Autodesk Inventor part; units mm, degrees
ref_plane "YZ Plane" through (0, 0, 0) normal (1, 0, 0) x (0, 1, 0)
ref_plane "XZ Plane" through (0, 0, 0) normal (0, 1, 0) x (-1, 0, 0)
ref_plane "XY Plane" through (0, 0, 0) normal (0, 0, 1) x (1, 0, 0)
sketch "Sketch1" plane through (0, 0, 0) normal (0, 0, 1) x (1, 0, 0)
  circle A0 centre (0, 0) radius 2.3813
  circle A1 centre (0, 0) radius 6.35
  dimension "d0" = 4.7625
  dimension "d1" = 12.7
extrude "Extrusion1" add sketch "Sketch1" along normal mid plane 4.9784
chamfer "Chamfer1" distance 0.1984 angle 45 4 edges at (-6.35, 0, 2.4892) (-2.3813, 0, 2.4892) (-6.35, 0, -2.4892) (-2.3813, 0, -2.4892)
sketch "Sketch2" plane through (0, 0, 0) normal (0, 1, 0) x (-1, 0, 0)
  line L0 (-6.1516, 2.4892) -> (6.1516, 2.4892)
  line L1 (2.5797, 2.4892) -> (-2.5797, 2.4892)
  line L2 (-5.5626, 2.4892) -> (-3.1686, 2.4892)
  line L3 (-3.1686, 2.4892) -> (-3.1686, 2.1082)
  line L4 (-3.1686, 2.1082) -> (-5.5626, 2.1082)
  line L5 (-5.5626, 2.1082) -> (-5.5626, 2.4892)
  line L6 (-6.35, -2.2908) -> (-6.35, 2.2908)
  line L7 (-2.3813, -2.2908) -> (-2.3813, 2.2908)
  line L8 (0, 0) -> (0, 3.7082)
  dimension "d7" = 0.381
  dimension "d8" = 0.7874
  dimension "d9" = 0.7874
revolve "Revolution1" cut sketch "Sketch2" angle 360 about axis through (0, 0, 0) along (0, 0, 1)
mirror "Mirror1" about plane through (0, 0, 0) normal (0, 0, 1) of "Revolution1"
equation "\"d9\" = d8"
properties part number "Homemade_bearing"
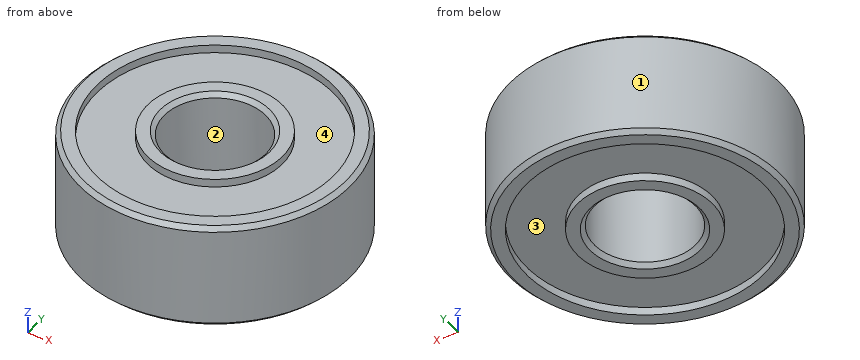
Verification items for the finished model (mm, model axes). Face numbers are marked on the shaded views. A direction names the side the tool comes from. Round coordinates to 2 decimals unless told otherwise and drop trailing zeros. Write each loop counter-clockwise with the first axis right and the second up, starting at its lowest first coordinate (ties: lowest second). Pieces come first, ordered by that corner, then holes. Notation, with made-up numbers: (65.25, -27) -> (100.25, -27) arc R14 ccw to (100.25, -5) -> close; hole circle Ø5 at (-13, 84). An arc over 180 degrees is marked (long way). Write each question's results on one line, items separated by ' | '. Start each with the question number.
1. Draft check along X on the marked faces 1 and 2. Enter one of: +X half, -X half, draft (parallel to the pull), parting line (faces both ways), or undercut.
2. Set-up check for the marked faces 3 and 4: record each of +Z, -Z, +X, -X, +Y, -Y from which the full face is reachable in a straight line by a thin tool's end or side.
3. Cross-section at C-C (z = -0.4). Enter the section's corners in (x, y), then the cut area to 3 significant figures.
4. Material ranges on probe 1 along Y at (x, z) = (0, -0.3); probe 2 along X at (y, z) = (-1.75, 1.4); probe 3 along X at (y, z) = (-1.25, -0.2), recorded low to high. Write a range as from..to.
Solutions:
1) face 1: parting line | face 2: undercut
2) face 3: -Z | face 4: +Z
3) outline: circle Ø12.7 at (0, 0); hole circle Ø4.76 at (0, 0) | area: 109 mm2
4) probe 1: y = -6.35..-2.38, 2.38..6.35 | probe 2: x = -6.1..-1.61, 1.61..6.1 | probe 3: x = -6.23..-2.03, 2.03..6.23
